Geometry: final body of the model. Coordinates: model frame, mm. Face numbers are marked on the shaded views. A direction names the side the tool comes from. Give positions to 0.01 mm unless a question says otherwise; leave off trailing zeros. Order: outer loops, then holes, each group sorted by start corner. A loop starts at its lowest first (then second) coordinate and runs counter-clockwise, first axis right, second up. Notation, with made-up numbers: M 89,7.5 L 93,7.5 A34 ccw 93,40.5 Z; hole C -15.5,1.25 d8. An arc over 180 degrees is marked long. One line per item, written item: value. Start each with the question number.
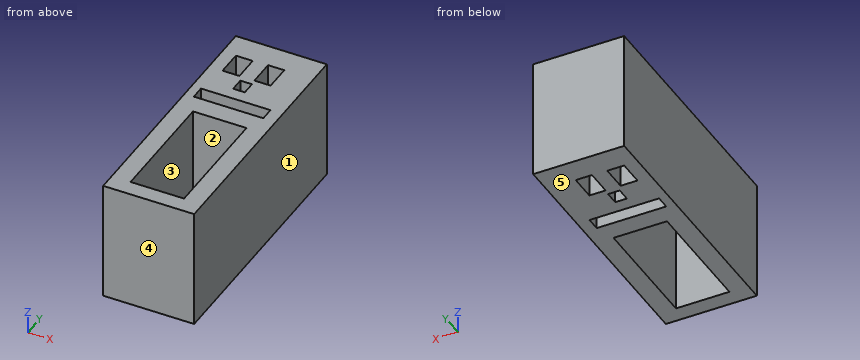
```python
from build123d import *

# Parameters (mm, degrees)
F0_W     = 22.498419
F0_H     = 50.058983
F0_W_2   = 29.24906
F0_H_2   = 5.740468
F0_W_3   = 7.107251
F0_H_3   = 10.660874
F1_DEPTH = 50.8


with BuildPart() as f1:
    # F0 (on Top) → F1 (new body)
    with BuildSketch(Plane.XY):
        Polygon((-21.644898, 52.593466), (-59.914693, 52.593466), (-59.914693, 39.472394), (-59.914693, 34.825347), (-59.914693, 6.66971), (-59.914693, -53.741902), (-56.087717, -53.741902), (-26.5653, -53.741902), (-21.644898, -53.741902), (-21.644898, 6.66971), (-21.644898, 34.825347), (-21.644898, 39.472394), align=None)
        with Locations((-40.778385, -21.795344)):
            Rectangle(F0_W, F0_H, mode=Mode.SUBTRACT)
        with Locations((-41.463187, 14.460347)):
            Rectangle(F0_W_2, F0_H_2, mode=Mode.SUBTRACT)
        Polygon((-45.426842, 22.797696), (-45.426842, 28.538166), (-40.600547, 28.538166), (-40.506441, 28.538166), (-40.506441, 22.797696), align=None, mode=Mode.SUBTRACT)
        with Locations((-50.6206, 36.328803)):
            Rectangle(F0_W_3, F0_H_3, mode=Mode.SUBTRACT)
        Polygon((-40.779795, 39.472394), (-40.779795, 41.932594), (-33.945903, 41.932594), (-33.945903, 30.998366), (-40.640878, 30.998366), (-40.779795, 30.998366), align=None, mode=Mode.SUBTRACT)
    extrude(amount=F1_DEPTH)


solid = f1.part
```
Q1. Section query D-D on x = -50.5. Return loops of the section in (y, z), and give its area (3 significant figures).
Q2. Mould query, pull axis Y, two halves, no side actions, for the marked faces 3, 4 and 5. Classes: +Y half, -Y half, draft (parallel to the pull), parting line (faces both ways), or undercut.
Q3. Ray query, line 1 along Y through (x, z) = (-36, 34); line 2 along Y through (x, z) = (-52.5, 7); line 3 along Y through (x, z) = (-47, 14). Return the intervals inside material, ascending. Write a range as [from, to].
Q4. Section query B-B on z = 12. Return loops of the section in (x, y), and give its area (3 significant figures).
Q5. Section query A-A on x = -35. Return loops of the section in (y, z).
Q6. Section query C-C on y = -40. Return loops of the section in (x, z).
Q7. Set-up query: the marked faces 1 and 2. Return all of +Z, -Z, +X, -X, +Y, -Y with unobstructed straight access to the full face (end or side cutting, diameter ignored); none if empty.
Results below:
1. outline: M -53.74,0 L -46.82,0 L -46.82,50.8 L -53.74,50.8 Z; M 3.23,0 L 11.59,0 L 11.59,50.8 L 3.23,50.8 Z; M 17.33,0 L 31,0 L 31,50.8 L 17.33,50.8 Z; M 41.66,0 L 52.59,0 L 52.59,50.8 L 41.66,50.8 Z
1. area: 2,030 mm2
2. face 3: undercut
2. face 4: -Y half
2. face 5: draft
3. line 1: [-53.74, -46.82], [3.23, 11.59], [17.33, 31], [41.93, 52.59]
3. line 2: [-53.74, 11.59], [17.33, 31], [41.66, 52.59]
3. line 3: [-53.74, -46.82], [3.23, 11.59], [17.33, 52.59]
4. outline: M -59.91,-53.74 L -21.64,-53.74 L -21.64,52.59 L -59.91,52.59 Z; hole M -56.09,11.59 L -26.84,11.59 L -26.84,17.33 L -56.09,17.33 Z; hole M -54.17,31 L -47.07,31 L -47.07,41.66 L -54.17,41.66 Z; hole M -52.03,-46.82 L -29.53,-46.82 L -29.53,3.23 L -52.03,3.23 Z; hole M -45.43,22.8 L -40.51,22.8 L -40.51,28.54 L -45.43,28.54 Z; hole M -40.78,31 L -33.95,31 L -33.95,41.93 L -40.78,41.93 Z
4. area: 2,600 mm2
5. outline: M -53.74,0 L -46.82,0 L -46.82,50.8 L -53.74,50.8 Z; M 3.23,0 L 11.59,0 L 11.59,50.8 L 3.23,50.8 Z; M 17.33,0 L 31,0 L 31,50.8 L 17.33,50.8 Z; M 41.93,0 L 52.59,0 L 52.59,50.8 L 41.93,50.8 Z
6. outline: M -59.91,0 L -52.03,0 L -52.03,50.8 L -59.91,50.8 Z; M -29.53,0 L -21.64,0 L -21.64,50.8 L -29.53,50.8 Z
7. face 1: +Z, -Z, +X, +Y, -Y
7. face 2: +Z, -Z
